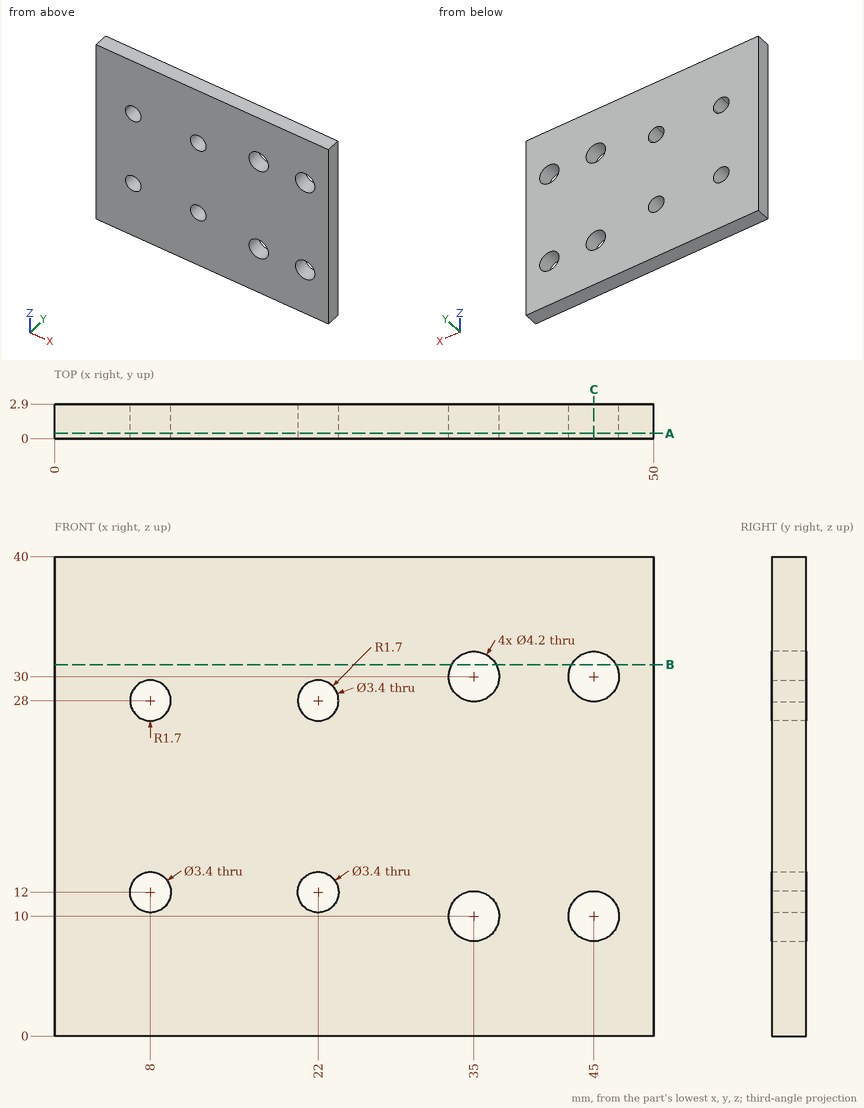
Check sheet for the drawn part. Datum: minimum x, y, z corner. Units: mm. Round coordinates to 2 decimals unless told otherwise and drop trailing zeros. Loops run counter-clockwise (first coordinate to the right, second up) from the corner with the lowest first, then second, coordinate; pieces in that order, holes last. Notation, with made-up numbers: (-27.5, 41.5) - (21.5, 41.5) arc R23 cw to (21.5, 64.5) - close; hole circle Ø6 at (-36.75, -18). An arc over 180 degrees is marked (long way). Write each question's results on one line, items separated by ' | '. Start each with the question number.
Q1. Cross-section at C-C on x = 45. Enter the section's corners in (y, z).
Q2. Thickness scan on line 1 (X direction, y = 1.35, z = 10); line 2 (Z direction, x = 22, y = 1.05); line 3 (Z direction, x = 34.5, y = 1.75). Record the ranges inside material, lowest first. Write a range as [from, to].
Q3. Cross-section at B-B on z = 31. Enter the section's corners in (x, y), and give its area (3 significant figures).
Q4. Cross-section at A-A on y = 0.45. State how many separate pieces and enclosed holes the cut face has, and give its area (3 significant figures).
Q5. Gauge pin test, flat end, axial feed: P1, Ø4, axis at x = 22, z = 12, coming from the +Y side. Record the tip position at first contact, or that the pin passes through.
Answers below:
1) outline: (0, 0) - (2.9, 0) - (2.9, 7.9) - (0, 7.9) - close; (0, 12.1) - (2.9, 12.1) - (2.9, 27.9) - (0, 27.9) - close; (0, 32.1) - (2.9, 32.1) - (2.9, 40) - (0, 40) - close
2) line 1: x = [0, 32.9], [37.1, 42.9], [47.1, 50] | line 2: z = [0, 10.3], [13.7, 26.3], [29.7, 40] | line 3: z = [0, 7.96], [12.04, 27.96], [32.04, 40]
3) outline: (0, 0) - (33.15, 0) - (33.15, 2.9) - (0, 2.9) - close; (36.85, 0) - (43.15, 0) - (43.15, 2.9) - (36.85, 2.9) - close; (46.85, 0) - (50, 0) - (50, 2.9) - (46.85, 2.9) - close | area: 124 mm²
4) separate pieces: 1 | enclosed holes: 8 | area: 1,910 mm²
5) P1: stops at y = 2.9
